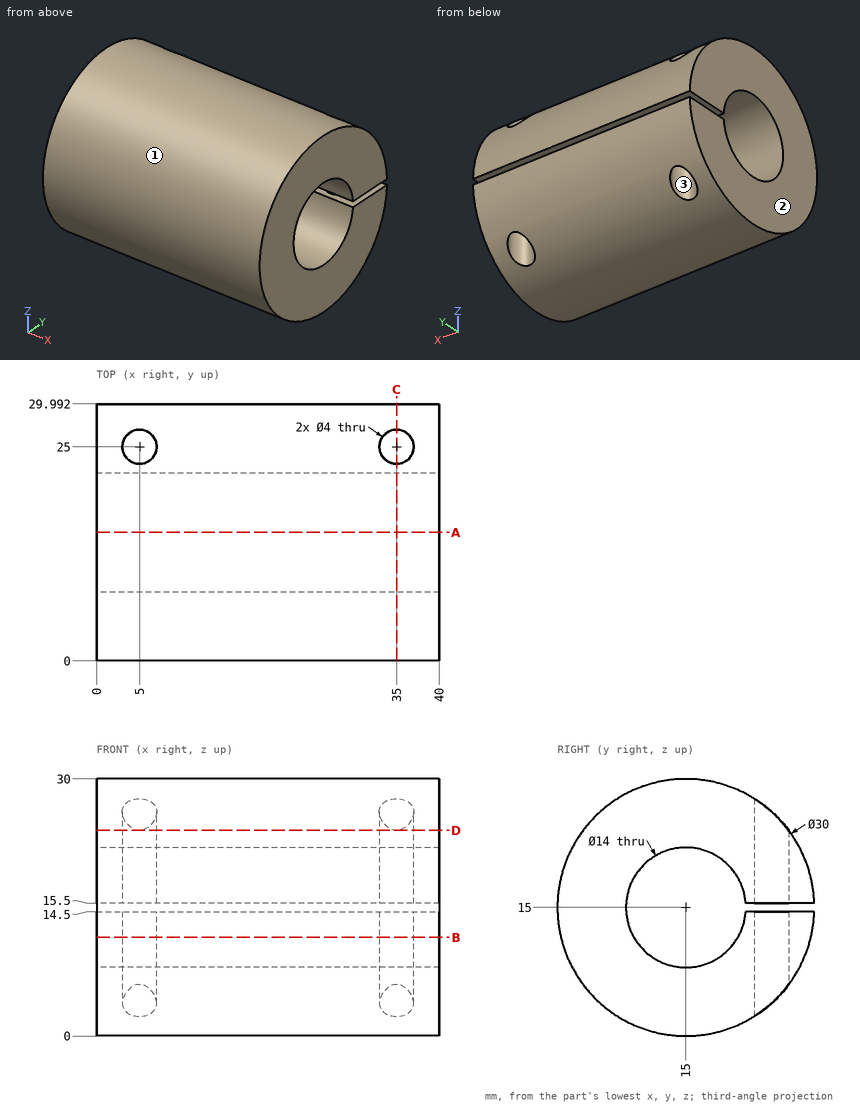
Design review of the part shown in the three views and the two pictorial views. Dimensions are in mm from the part's minimum x, y and z. Round coordinates to 2 decimals unless told otherwise and drop trailing zeros. Order: outer loops, then holes, each group sorted by start corner. A loop starts at its lowest first (then second) coordinate and runs counter-clockwise, first axis right, second up.
(1) Take a section at D-D, the plane z = 24. State the section outline as (x, y) points.
Working result:
outline: (0, 3) - (40, 3) - (40, 27) - (0, 27) - close; hole circle Ø4 at (5, 25); hole circle Ø4 at (35, 25)
(2) Take a section at A-A, the plane y = 15. State the section outline as (x, z) points.
Working result:
outline: (0, 0) - (40, 0) - (40, 8) - (0, 8) - close; (0, 22) - (40, 22) - (40, 30) - (0, 30) - close
(3) Take a section at C-C, the plane x = 35. State the section outline as (y, z) points.
Working result:
outline: (21.98, 14.5) arc R7 cw (long way) to (21.98, 15.5) - (23, 15.5) - (23, 27.69) arc R15 ccw (long way) to (23, 2.31) - (23, 14.5) - close; (27, 6) arc R15 ccw to (29.99, 14.5) - (27, 14.5) - close; (27, 15.5) - (29.99, 15.5) arc R15 ccw to (27, 24) - close
(4) Mouldability with a two-part tool opening along Y and no side actions: class the marked faces 1, 2 and 3 as released by +Y, released by -Y, zero draft, split by the parting line, or undercut.
Working result:
face 1: split by the parting line
face 2: zero draft
face 3: undercut
(5) Wall thickness on L1, parallel to Y at x = 5, z = 11 (1 decimal); L2, parallel to Y at x = 35, z = 11.75 (1 decimal); L3, parallel to Z at x = 21, y = 14.25: over which ranges is each line inside the solid? List them lowest first.
Working result:
L1: y = 0.5 to 9.3, 20.7 to 23, 27 to 29.5
L2: y = 0.4 to 8.8, 21.2 to 23, 27 to 29.6
L3: z = 0.02 to 8.04, 21.96 to 29.98
(6) For P1, Ø12, axis at x = 17, z = 26.5, coming from the -Y side (1 decimal); P2, Ø4.5, axis at x = 5, y = 25, coming from the -Z side; P3, Ø10, axis at x = 19, z = 5, coming from the -Y side; P4, Ø2.5, axis at x = 35, y = 25, coming from the -Z side, all flat-tipped, find the tip position at first contact; note any pin that passes through.
Working result:
P1: stops at y = 1
P2: stops at z = 2.16
P3: stops at y = 0.86
P4: passes through
(7) Take a section at B-B, the plane z = 11.5. State the section outline as (x, y) points, plus the area to 3 significant figures.
Working result:
outline: (0, 0.41) - (40, 0.41) - (40, 8.94) - (0, 8.94) - close; (0, 21.06) - (40, 21.06) - (40, 29.59) - (0, 29.59) - close; hole circle Ø4 at (5, 25); hole circle Ø4 at (35, 25)
area: 657 mm2
